CAD build for the part. Positions are in the model's coordinates, mm. A direction names the side the tool comes from. Give positions to 0.01 mm unless a question says otherwise; leave off trailing zeros. Write each loop counter-clockwise with the first axis right and the second up, starting at its lowest first coordinate (ties: lowest second). Pieces come first, ordered by that corner, then holes. Notation, with made-up numbers: (52.25, -17) - (67.25, -17) arc R24 ccw to (67.25, -6) - close; hole circle Ø10 at (-36.75, -36). An arc over 180 degrees is marked (long way). Write item = value, one per line. Start each with the question number.
```python
from build123d import *

# Parameters (mm, degrees)
F1_DEPTH = 88.9
F3_W     = 72.389998
F3_H     = 88.9
F4_DEPTH = 20
F5_W     = 15
F5_H     = 76.5
F6_DEPTH = 40
F7_W     = 10.8
F7_H     = 12.7
F7_W_2   = 40
F8_DEPTH = 110.672824


with BuildPart() as f1:
    # F0 (on Top) → F1 (new body)
    with BuildSketch(Plane.XY):
        with BuildLine():
            ThreePointArc((43.122277, 40.17818), (-11.239462, 13.991304), (-50.049547, -32.211818))
            Line((-50.049547, -32.211818), (43.122277, -32.211818))
            Line((43.122277, -32.211818), (43.122277, 40.17818))
        make_face()
    extrude(amount=F1_DEPTH)

    # F3 (on face) → F4 (join)
    with BuildSketch(Plane.YZ.offset(43.122277)):
        with Locations((3.983181, 44.45)):
            Rectangle(F3_W, F3_H)
    extrude(amount=F4_DEPTH)

    # F5 (on face) → F6 (cut)
    with BuildSketch(Plane(origin=(0, 40.17818, 0), x_dir=(-1, 0, 0), z_dir=(0, 1, 0))):
        with Locations((-53.122277, 44.45)):
            Rectangle(F5_W, F5_H)
    extrude(amount=-F6_DEPTH, mode=Mode.SUBTRACT)

    # F7 (on face) → F8 (cut, through all)
    with BuildSketch(Plane(origin=(60.622277, 0, 0), x_dir=(0, -1, 0), z_dir=(-1, 0, 0))):
        with Locations((5.22182, 15.852)):
            Rectangle(F7_W, F7_H)
        with Locations((5.22182, 34.902)):
            Rectangle(F7_W, F7_H)
        with Locations((5.22182, 53.952)):
            Rectangle(F7_W, F7_H)
        with Locations((5.22182, 73.048)):
            Rectangle(F7_W, F7_H)
        with Locations((-20.17818, 15.852)):
            Rectangle(F7_W_2, F7_H)
        with Locations((-20.17818, 34.902)):
            Rectangle(F7_W_2, F7_H)
        with Locations((-20.17818, 53.952)):
            Rectangle(F7_W_2, F7_H)
        with Locations((-20.17818, 73.048)):
            Rectangle(F7_W_2, F7_H)
    extrude(amount=F8_DEPTH, mode=Mode.SUBTRACT)


solid = f1.part
```
1. Cut at A-A (y = 10.5). Give the cut face in (x, z).
2. Cut at C-C (z = 25). Give the cut face in (x, y), then the cut area to 3 significant figures.
3. Cut at B-B (x = 1.5). Give the cut face in (y, z).
4. Pin check, flat tips, straight feed: pin 1 Ø10 at (x, z) = (12, 15) entering from +Y; pin 2 Ø1.7 at (x, z) = (55.5, 81.5) entering from +Y; pin 3 Ø8 at (y, z) = (-19, 42) entering from -X. Stop position of each tip, or through.
5. Tool access for faces 5 (the flat face through (44, 40.178, 25)), 6 (the flat face through (53, 20, 82.7)), 7 (the flat face through (24, 9, 79.398)): list every direction of +Z, -Z, +X, -X, +Y, -Y with a clear straight run to the whole face (end or side of a thin tool).
6. Wall check: line 1 along Z through (x, y) = (17, 10.5); line 2 along X through (y, z) = (8, 13); line 3 along Y through (x, z) = (10, 33.5). Give the ranges that are in metal, low to high.
7. Cut at D-D (y = -2). Give the cut face in (x, z), then the cut area to 3 significant figures.
8. Mould opens along X. For faces 1 (the flat face through (53, 0.178, 44)), 2 (the cylindrical face through (-20.881, 5.795, 43.828)), 3 (the flat face through (13, -10.622, 54)), 4 (the flat face through (53, 0.178, 81)) say: +X half, -X half, draft (parallel to the pull), parting line (faces both ways), or undercut.
Output:
q1.outline = (-15.56, 0) - (63.12, 0) - (63.12, 88.9) - (-15.56, 88.9) - (-15.56, 79.4) - (45.62, 79.4) - (45.62, 82.7) - (60.62, 82.7) - (60.62, 6.2) - (45.62, 6.2) - (45.62, 9.5) - (-15.56, 9.5) - close; (-15.56, 22.2) - (45.62, 22.2) - (45.62, 28.55) - (-15.56, 28.55) - close; (-15.56, 41.25) - (45.62, 41.25) - (45.62, 47.6) - (-15.56, 47.6) - close; (-15.56, 60.3) - (45.62, 60.3) - (45.62, 66.7) - (-15.56, 66.7) - close
q2.outline = (-50.05, -32.21) - (63.12, -32.21) - (63.12, 40.18) - (60.62, 40.18) - (60.62, 0.18) - (45.62, 0.18) - (45.62, 40.18) - (43.12, 40.18) arc R143.64 ccw to start
q2.area = 5,230 mm2
q3.outline = (-32.21, 0) - (22.83, 0) - (22.83, 9.5) - (-10.62, 9.5) - (-10.62, 22.2) - (22.83, 22.2) - (22.83, 28.55) - (-10.62, 28.55) - (-10.62, 41.25) - (22.83, 41.25) - (22.83, 47.6) - (-10.62, 47.6) - (-10.62, 60.3) - (22.83, 60.3) - (22.83, 66.7) - (-10.62, 66.7) - (-10.62, 79.4) - (22.83, 79.4) - (22.83, 88.9) - (-32.21, 88.9) - close
q4.pin_1 = -10.62
q4.pin_2 = 0.18
q4.pin_3 = -44.73
q5.face_5 = +Z, -Z, +X, -X, +Y
q5.face_6 = +Y
q5.face_7 = -X, +Y
q6.line_1 = 0 to 9.5, 22.2 to 28.55, 41.25 to 47.6, 60.3 to 66.7, 79.4 to 88.9
q6.line_2 = 60.62 to 63.12
q6.line_3 = -32.21 to -10.62
q7.outline = (-28.65, 0) - (63.12, 0) - (63.12, 88.9) - (-28.65, 88.9) - (-28.65, 79.4) - (60.62, 79.4) - (60.62, 66.7) - (-28.65, 66.7) - (-28.65, 60.3) - (60.62, 60.3) - (60.62, 47.6) - (-28.65, 47.6) - (-28.65, 41.25) - (60.62, 41.25) - (60.62, 28.55) - (-28.65, 28.55) - (-28.65, 22.2) - (60.62, 22.2) - (60.62, 9.5) - (-28.65, 9.5) - close
q7.area = 3,620 mm2
q8.face_1 = undercut
q8.face_2 = -X half
q8.face_3 = draft
q8.face_4 = undercut
